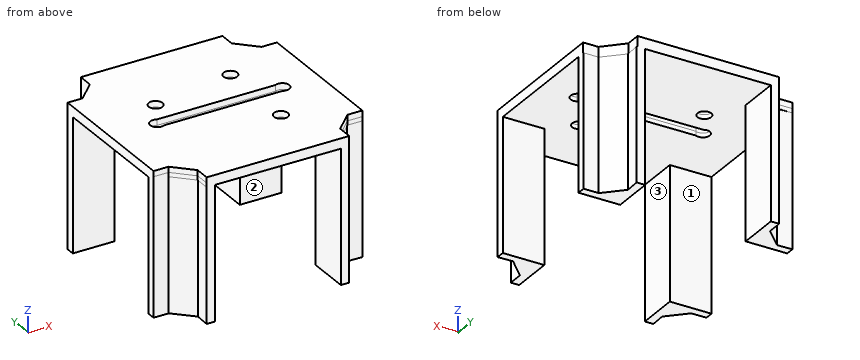
Autodesk Inventor part; units mm, degrees
ref_plane "Work Plane1" through (-29.1, -14.5, 2.4) normal (0, 0, -1) x (0, 1, 0)
ref_plane "Work Plane2" through (-13.8999, -10.5497, 2.25) normal (0, 0, -1) x (0, 1, 0)
ref_plane "Work Plane4" through (-17.3325, -17.0101, 2.3331) normal (0.0023, 0.0023, -1) x (0, 1, 0.0023)
ref_plane "Work Plane1" through (-29.1, -14.5, 2.4) normal (0, 0, -1) x (0, 1, 0)
ref_plane "Work Plane2" through (-13.8999, -10.5497, 2.25) normal (0, 0, -1) x (0, 1, 0)
ref_plane "Work Plane4" through (-17.3325, -17.0101, 2.3331) normal (0.0023, 0.0023, -1) x (0, 1, 0.0023)
sketch "Sketch1" plane through (0, 0, 0) normal (0, 0, 1) x (1, 0, 0)
  line L0 (-34.86, 0) -> (34.86, 0) construction
  line L1 (0, -34.86) -> (0, 34.86) construction
  line L2 (0, 0) -> (11.1575, 11.1575) construction
  line L3 (0, 0) -> (15.7791, 0) construction
  line L4 (0, 24.9) -> (16.8009, 24.9)
  line L5 (16.8009, 24.9) -> (16.8009, 21.2415)
  line L6 (16.8009, 21.2415) -> (19.0212, 19.0212)
  line L7 (24.9, 0) -> (24.9, 16.8009)
  line L8 (24.9, 16.8009) -> (21.2415, 16.8009)
  line L9 (21.2415, 16.8009) -> (19.0212, 19.0212)
  line L10 (0, -24.9) -> (16.8009, -24.9)
  line L11 (16.8009, -24.9) -> (16.8009, -21.2415)
  line L12 (16.8009, -21.2415) -> (19.0212, -19.0212)
  line L13 (24.9, 0) -> (24.9, -16.8009)
  line L14 (24.9, -16.8009) -> (21.2415, -16.8009)
  line L15 (21.2415, -16.8009) -> (19.0212, -19.0212)
  line L16 (0, 24.9) -> (-16.8009, 24.9)
  line L17 (-16.8009, 24.9) -> (-16.8009, 21.2415)
  line L18 (-16.8009, 21.2415) -> (-19.0212, 19.0212)
  line L19 (-24.9, 16.8009) -> (-21.2415, 16.8009)
  line L20 (-21.2415, 16.8009) -> (-19.0212, 19.0212)
  line L21 (0, -24.9) -> (-16.8009, -24.9)
  line L22 (-16.8009, -24.9) -> (-16.8009, -21.2415)
  line L23 (-16.8009, -21.2415) -> (-19.0212, -19.0212)
  line L24 (-21.2415, -16.8009) -> (-19.0212, -19.0212)
  line L25 (-24.9, -16.8009) -> (-21.2415, -16.8009)
  line L26 (-24.9, 0) -> (-24.9, -16.8009)
  line L27 (-24.9, 0) -> (-24.9, 16.8009)
  circle A0 centre (0, 0) radius 10
  dimension "d0" = 45
  dimension "d2" = 24.9
  dimension "d3" = 3.14
  dimension "d4" = 26.9
  dimension "d5" = 20
extrude "Extrusion1" add sketch "Sketch1" along normal blind 1 contours L4 L5 L6 L9 L8 L7 L13 L14 L15 L12 L11 L10 L21 L22 L23 L24 L25 L26 L27 L19 L20 L18 L17 L16 | A0
sketch "Sketch5" plane through (0, 0, 0) normal (0, 0, -1) x (-1, 0, 0)
  circle A0 centre (-9.7, 10) radius 1.4
  circle A1 centre (-9.7, -10) radius 1.4
  circle A2 centre (13.8, 0) radius 1.4
  circle A3 centre (-10, 6.9) radius 0.75
  circle A4 centre (10, 6.9) radius 1.25
  point P0 (0, 0)
hole "Hole1" at (-13.8, 0, 0) at (9.7, -10, 0) at (-10, 6.9, 0) at (9.7, 10, 0) direction (0, 0, 1) diameter 3.3 depth 12 tip angle 118
sketch "Skizze6" plane through (-16.8009, 24.9, 1) normal (0, 0, 1) x (1, 0, 0)
  circle A0 centre (6.8009, -18) radius 1.65 construction
  circle A1 centre (3.0009, -24.9) radius 1.65 construction
  circle A2 centre (26.5009, -34.9) radius 1.65 construction
  circle A3 centre (26.5009, -14.9) radius 1.65 construction
  line L0 (33.6017, -3.6585) -> (33.6017, 0)
  line L1 (33.6017, 0) -> (0, 0) construction
  line L2 (0, 0) -> (0, -3.6585)
  line L3 (0, -3.6585) -> (-4.4406, -8.0991)
  line L4 (-4.4406, -8.0991) -> (-8.0991, -8.0991)
  line L5 (-8.0991, -8.0991) -> (-8.0991, -41.7009) construction
  line L6 (-8.0991, -41.7009) -> (-4.4406, -41.7009)
  line L7 (-4.4406, -41.7009) -> (0, -46.1415)
  line L8 (0, -46.1415) -> (0, -49.8)
  line L9 (0, -49.8) -> (33.6017, -49.8) construction
  line L10 (33.6017, -49.8) -> (33.6017, -46.1415)
  line L11 (33.6017, -46.1415) -> (38.0423, -41.7009)
  line L12 (38.0423, -41.7009) -> (41.7009, -41.7009)
  line L13 (41.7009, -41.7009) -> (41.7009, -8.0991) construction
  line L14 (41.7009, -8.0991) -> (38.0423, -8.0991)
  line L15 (38.0423, -8.0991) -> (33.6017, -3.6585)
  line L16 (-0.2, 0.2) -> (33.8017, 0.2) construction
  line L17 (33.8017, 0.2) -> (33.8017, -3.5757)
  line L18 (33.8017, -3.5757) -> (38.1252, -7.8991)
  line L19 (38.1252, -7.8991) -> (41.9009, -7.8991)
  line L20 (41.9009, -7.8991) -> (41.9009, -41.9009) construction
  line L21 (41.9009, -41.9009) -> (38.1252, -41.9009)
  line L22 (38.1252, -41.9009) -> (33.8017, -46.2243)
  line L23 (33.8017, -46.2243) -> (33.8017, -50)
  line L24 (33.8017, -50) -> (-0.2, -50) construction
  line L25 (-0.2, -50) -> (-0.2, -46.2243)
  line L26 (-0.2, -46.2243) -> (-4.5235, -41.9009)
  line L27 (-4.5235, -41.9009) -> (-8.2991, -41.9009)
  line L28 (-8.2991, -41.9009) -> (-8.2991, -7.8991) construction
  line L29 (-8.2991, -7.8991) -> (-4.5235, -7.8991)
  line L30 (-4.5235, -7.8991) -> (-0.2, -3.5757)
  line L31 (-0.2, -3.5757) -> (-0.2, 0.2)
  line L32 (-8.0991, -8.0991) -> (-8.0991, -7.8991)
  line L33 (0, 0) -> (-0.2, 0)
  line L34 (33.6017, 0) -> (33.8017, 0)
  line L35 (41.7009, -8.0991) -> (38.0423, -8.0991)
  line L36 (41.7009, -8.0991) -> (41.7009, -7.8991)
  line L37 (41.7009, -41.7009) -> (41.7009, -41.9009)
  line L38 (33.6017, -49.8) -> (33.8017, -49.8)
  line L39 (-8.0991, -41.7009) -> (-8.0991, -41.9009)
  line L40 (0, -49.8) -> (-0.2, -49.8)
  point P0 (16.8009, -24.9)
  dimension "d25" = 0.2
extrude "IM_offset" add sketch "Skizze6" against normal blind 1 contours L2 L3 L4 L32 L29 L30 L31 L33 | L6 L7 L8 L40 L25 L26 L27 L39 | L10 L11 L12 L37 L21 L22 L23 L38
sketch "Sketch7" plane through (-24.9, 16.9009, 1) normal (0, 0, 1) x (1, 0, 0)
  circle A0 centre (11.1, -16.9009) radius 1.65
  line L0 (11.1, -16.9009) -> (40.9762, -16.9009) construction
  line L1 (11.1, -18.3509) -> (40.9762, -18.3509)
  line L2 (40.9762, -15.4509) -> (11.1, -15.4509)
  arc A1 (11.1, -15.4509) -> (11.1, -18.3509) centre (11.1, -16.9009) ccw
  arc A2 (40.9762, -18.3509) -> (40.9762, -15.4509) centre (40.9762, -16.9009) ccw
  circle A3 centre (40.9762, -16.9009) radius 1.65
  point P0 (24.9, -16.9009)
  point P1 (26.0381, -16.9009)
  dimension "d28" = 2.9
extrude "Extrusion6" cut sketch "Sketch7" against normal blind 10 contours A0 L1 A1 L2 | A0 L2 A3 L1 | A3 L1 A2 L2 | L2 A2 L1 A3 picked at (11.65, -16.9009)
ref_plane "Work Plane3" through (-24.85, -16.97, -31.85) normal (0, 0, 1) x (1, 0, 0)
sketch "Sketch9" plane through (0, 0, 0) normal (0, 0, -1) x (-1, 0, 0)
  line L0 (21.2829, 16.9009) -> (17.0009, 21.2829)
  line L1 (17.0009, 21.2829) -> (17.0009, 24.9)
  line L2 (24.9, 17.0009) -> (21.2829, 16.9009)
  line L3 (24.9, -17.0009) -> (24.9, 17.0009)
  line L4 (17.0009, 24.9) -> (-16.8009, 24.9)
  line L5 (24.9, 14.96) -> (15.0009, 14.96)
  line L6 (15.0009, 14.96) -> (15.0009, 24.9)
  line L7 (15.0009, 24.9) -> (17.0009, 24.9)
  line L8 (24.9, 17.0009) -> (24.9, 14.96)
  line L9 (-16.9009, 21.2829) -> (-21.2829, 17.0009)
  line L10 (-21.2829, 17.0009) -> (-24.9, 17.0009)
  line L11 (-17.0009, 24.9) -> (-16.9009, 21.2829)
  line L12 (-14.96, 24.9) -> (-14.96, 15.0009)
  line L13 (-14.96, 15.0009) -> (-24.9, 15.0009)
  line L14 (-24.9, 15.0009) -> (-24.9, 17.0009)
  line L15 (-17.0009, 24.9) -> (-14.96, 24.9)
  line L16 (-21.2829, -16.9009) -> (-17.0009, -21.2829)
  line L17 (-17.0009, -21.2829) -> (-17.0009, -24.9)
  line L18 (-24.9, -17.0009) -> (-21.2829, -16.9009)
  line L19 (-24.9, -14.96) -> (-15.0009, -14.96)
  line L20 (-15.0009, -14.96) -> (-15.0009, -24.9)
  line L21 (-15.0009, -24.9) -> (-17.0009, -24.9)
  line L22 (-24.9, -17.0009) -> (-24.9, -14.96)
  line L23 (16.9009, -21.2829) -> (21.2829, -17.0009)
  line L24 (21.2829, -17.0009) -> (24.9, -17.0009)
  line L25 (17.0009, -24.9) -> (16.9009, -21.2829)
  line L26 (14.96, -24.9) -> (14.96, -15.0009)
  line L27 (14.96, -15.0009) -> (24.9, -15.0009)
  line L28 (24.9, -15.0009) -> (24.9, -17.0009)
  line L29 (17.0009, -24.9) -> (14.96, -24.9)
  point P0 (0, 0)
  dimension "d44" = 2
  dimension "d47" = 360
ref_plane "Work Plane5" through (-25.1325, -16.9302, -31.7852) normal (-0.0023, -0.0023, 1) x (1, 0, 0.0023)
extrude "Extrusion9" add sketch "Sketch9" along normal up to surface surface through (-25.1325, -16.9302, -31.7852) normal (-0.0023, -0.0023, 1)
ref_plane "Work Plane6" through (-16.5464, -17.0101, 2.3349) normal (0.0023, 0.0023, -1) x (0, 1, 0.0023)
sketch "Sketch11" plane through (0, 0, 1) normal (0, 0, 1) x (1, 0, 0)
  circle A0 centre (-10, 6.9) radius 1.65
  circle A1 centre (9.7, 10) radius 1.65
  circle A2 centre (9.7, -10) radius 1.65
  arc A3 (-13.0126, 1.45) -> (-13.0126, -1.45) centre (-13.8, 0) ccw
  line L0 (-13.0126, 1.45) -> (15.2888, 1.45)
  line L1 (15.2888, -1.45) -> (-13.0126, -1.45)
  arc A4 (15.2888, -1.45) -> (15.2888, 1.45) centre (16.0762, 0) ccw
  line L2 (16.8009, 24.9) -> (-17.0009, 24.9)
  line L3 (-17.0009, 24.9) -> (-17.0009, 21.3243)
  line L4 (-17.0009, 21.3243) -> (-21.3243, 17.0009)
  line L5 (-21.3243, 17.0009) -> (-24.9, 17.0009)
  line L6 (-24.9, 17.0009) -> (-24.9, -17.0009)
  line L7 (-24.9, -17.0009) -> (-21.3243, -17.0009)
  line L8 (-21.3243, -17.0009) -> (-17.0009, -21.3243)
  line L9 (-17.0009, -21.3243) -> (-17.0009, -24.9)
  line L10 (-17.0009, -24.9) -> (17.0009, -24.9)
  line L11 (17.0009, -24.9) -> (17.0009, -21.3243)
  line L12 (17.0009, -21.3243) -> (21.3243, -17.0009)
  line L13 (21.3243, -17.0009) -> (24.9, -17.0009)
  line L14 (24.9, -17.0009) -> (24.9, 16.8009)
  line L15 (24.9, 16.8009) -> (21.2415, 16.8009)
  line L16 (21.2415, 16.8009) -> (16.8009, 21.2415)
  line L17 (16.8009, 21.2415) -> (16.8009, 24.9)
  circle A5 centre (9.7, 10) radius 1.65
  circle A6 centre (9.7, -10) radius 1.65
  line L18 (-13.0126, 1.45) -> (15.2888, 1.45)
  arc A7 (15.2888, -1.45) -> (15.2888, 1.45) centre (16.0762, 0) ccw
  line L19 (15.2888, -1.45) -> (-13.0126, -1.45)
  arc A8 (-13.0126, 1.45) -> (-13.0126, -1.45) centre (-13.8, 0) ccw
  circle A9 centre (-10, 6.9) radius 1.65
  point P0 (0, 0)
ref_plane "Work Plane7" through (-24.4263, -24.8901, 2.298) normal (0.0023, 0.0023, -1) x (0, 1, 0.0023)
extrude "Extrusion11" add sketch "Sketch11" along normal up to surface surface through (-24.4263, -24.8901, 2.298) normal (0.0023, 0.0023, -1)
equation "\"BendRadius\" = Thickness"
equation "\"BendReliefWidth\" = Thickness"
equation "\"BendReliefDepth\" = 0.5 * Thickness"
equation "\"CornerReliefSize\" = 4 * Thickness"
equation "\"MinimumRemnant\" = 2 * Thickness"
equation "\"TransitionRadius\" = BendRadius"
equation "\"JacobiRadiusSize\" = Thickness"
equation "\"GapSize\" = Thickness"
properties part number "20_Cube_insert_AlliedVision_Alvium_v3"
Design review of the part built by this model. Coordinates are the model's own, in mm. Face numbers are marked on the shaded views. Coordinates: 2 decimals unless noted, no trailing zeros. Loops run counter-clockwise (first coordinate to the right, second up) from the corner with the lowest first, then second, coordinate; pieces in that order, holes last. Notation, with made-up numbers: M -14,0.25 L 6,0.25 A10 cw 6,18.25 Z; hole C -31,25 d11. An arc over 180 degrees is marked long. Use one line per item in the form item = value.
(1) For line 1 along Y through (x, z) = (9.7, 1.55); line 2 along X through (y, z) = (0, 1); line 3 along X through (y, z) = (-10, 0.7), list the stretches that pass through material, from the lowest coordinate up. Write a range as from..to.
Return value:
line_1 = -24.9..-11.65, -8.35..-1.45, 1.45..8.35, 11.65..24.9
line_2 = -24.9..-15.45, 17.73..24.9
line_3 = -24.9..8.05, 11.35..24.9
(2) Consider section B-B (x = 5). Write out the cut boundary in (y, z), and give its area (3 significant figures).
Return value:
outline = M -24.9,0 L -1.45,0 L -1.45,2.42 L -24.9,2.37 Z; M 1.45,0 L 24.9,0 L 24.9,2.48 L 1.45,2.43 Z
area = 114 mm2
(3) Consider section A-A (z = -23). Write out the cut boundary in (x, y).
Return value:
outline = M -24.9,-17 L -21.28,-17 L -16.9,-21.28 L -17,-24.9 L -14.96,-24.9 L -14.96,-15 L -24.9,-15 Z; M -24.9,14.96 L -15,14.96 L -15,24.9 L -17,24.9 L -17,21.28 L -21.28,16.9 L -24.9,17 Z; M 14.96,15 L 24.9,15 L 24.9,17 L 21.28,17 L 16.9,21.28 L 17,24.9 L 14.96,24.9 Z; M 15,-24.9 L 17,-24.9 L 17,-21.28 L 21.28,-16.9 L 24.9,-17 L 24.9,-14.96 L 15,-14.96 Z
(4) Clearance check with flat-ended pins moving along their axes: P1, Ø1.8, axis at x = -22.5, z = -15.5, coming from the -Y side; P2, Ø1.5, axis at x = -22.5, z = 1.5, coming from the +Y side; P3, Ø3, axis at y = 22.5, z = -8, coming from the -X side. State where each tip first meets the part, or that it passes through.
Return value:
P1 = -17
P2 = 17
P3 = -17.28
(5) Consider section C-C (y = -10). Write out the cut boundary in (x, z).
Return value:
outline = M -24.9,0 L 8.05,0 L 8.05,2.41 L -24.9,2.33 Z; M 11.35,0 L 24.9,0 L 24.9,2.45 L 11.35,2.41 Z
(6) Draft analysis for pull direction Y (two halves, no side actions). For the marked faces 1, 2 and 3, state which applies: pulls with the +Y half, pulls with the -Y half, needs draft (parallel to the pull), parting line crosses it, or undercut.
Return value:
face_1 = undercut
face_2 = undercut
face_3 = needs draft
(7) Consider section D-D (x = -10). Write out the cut boundary in (y, z), and give its area (3 significant figures).
Return value:
outline = M -24.9,0 L -1.45,0 L -1.45,2.39 L -24.9,2.33 Z; M 1.45,0 L 5.25,0 L 5.25,2.4 L 1.45,2.39 Z; M 8.55,0 L 24.9,0 L 24.9,2.45 L 8.55,2.41 Z
area = 104 mm2
